from build123d import *

# Parameters (mm, degrees)
TAPPED_HOLE1_D     = 6.8
SKETCH4_W          = 9.5
SKETCH4_H          = 1.5
CUT_EXTRUDE1_DEPTH = 12


with BuildPart() as part:
    # Sketch1 → Revolve1 (revolve)
    with BuildSketch(Plane(origin=(0, 0, 0), x_dir=(0, 0, -1), z_dir=(1, 0, 0))):
        Polygon((-4.75, -13.8), (-4.75, -1.4), (-4.65, -1.4), (-4.65, -1.3), (-5.55, -1.3), (-5.55, 0), (-3.25, 0), (-3.25, -14.3), (-4.461324865, -14.3), align=None)
    revolve(axis=Axis((0, 0, 0), (0, -1, 0)))

    # Tapped Hole1 (through all)
    with Locations(Plane(origin=(0, 0, 0), x_dir=(1, 0, 0), z_dir=(0, 1, 0))):
        with Locations((0, 0)):
            Hole(TAPPED_HOLE1_D / 2)

    # Sketch4 → Cut-Extrude1 (cut)
    with BuildSketch(Plane.XZ.offset(14.3)):
        Rectangle(SKETCH4_W, SKETCH4_H)
    extrude(amount=-CUT_EXTRUDE1_DEPTH, mode=Mode.SUBTRACT)


solid = part.part
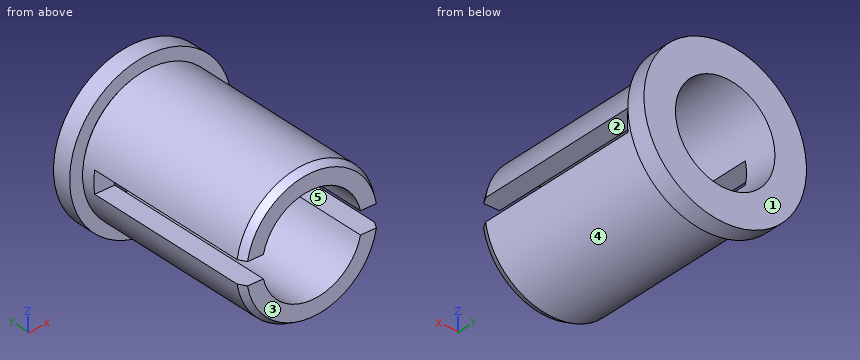
Geometry: final body of the model. Coordinates: model frame, mm. Face numbers are marked on the shaded views. A direction names the side the tool comes from. Coordinates: 2 decimals unless noted, no trailing zeros. Order: outer loops, then holes, each group sorted by start corner. A loop starts at its lowest first (then second) coordinate and runs counter-clockwise, first axis right, second up.
(1) Section query A-A (x = 0). Return the cut outline in (y, z).
(2) Draft query along Z for the marked faces 3, 4 and 5. Return one class per face: pulls with the +Z half, pulls with the -Z half, needs draft (parallel to the pull), parting line crosses it, or undercut.
(3) First-contact query: pin 1 (4 mm diameter, centred on y = -9.5, z = 2, fed in from +X); pin 2 (6 mm diameter, centred on y = -12.5, z = -3, fed in from -X); pin 3 (1.1 mm diameter, centred on x = -4, y = -8.5, fed in from -Z). Flat tips, straight axial feed; report the tip coordinate or a pass-through.
(4) Section query D-D (y = -2). Return the cut outline in (x, z).
(5) Access query for the marked faces 1 and 2. Directions: +Z, -Z, +X, -X, +Y, -Y. A direction counts if a zero-diameter tool reaches every point of the face in a straight line with its end or side. Return the directions, or none.
(6) Section query B-B (z = 0). Return the cut outline in (x, y), plus the area to 3 significant figures.
(7) Material intervals for probe 1 along Z at (x, y) = (0, -10.75); probe 2 along Z at (x, y) = (1, -4.75); probe 3 along Y at (x, z) = (-3.75, 3.25), sorted ascending.
(8) Section query C-C (y = -3.75). Return the cut outline in (x, z), plus the area to 3 significant figures.
Solution:
1. outline: (-14.3, -4.46) - (-13.8, -4.75) - (-1.4, -4.75) - (-1.4, -4.65) - (-1.3, -4.65) - (-1.3, -5.55) - (0, -5.55) - (0, -3.4) - (-14.3, -3.4) - close; (-14.3, 3.4) - (0, 3.4) - (0, 5.55) - (-1.3, 5.55) - (-1.3, 4.65) - (-1.4, 4.65) - (-1.4, 4.75) - (-13.8, 4.75) - (-14.3, 4.46) - close
2. face 3: needs draft
2. face 4: parting line crosses it
2. face 5: undercut
3. pin 1: stops at x = 4.69
3. pin 2: stops at x = -4.69
3. pin 3: stops at z = -3.26
4. outline: circle Ø9.5 at (0, 0); hole circle Ø6.8 at (0, 0)
5. face 1: +Z, -Z, +X, -X, +Y
5. face 2: +X, -X, -Y
6. outline: (-5.55, -1.3) - (-4.65, -1.3) - (-4.65, -1.4) - (-4.75, -1.4) - (-4.75, -2.3) - (-3.4, -2.3) - (-3.4, 0) - (-5.55, 0) - close; (3.4, -2.3) - (4.75, -2.3) - (4.75, -1.4) - (4.65, -1.4) - (4.65, -1.3) - (5.55, -1.3) - (5.55, 0) - (3.4, 0) - close
6. area: 8.27 mm2
7. probe 1: z = -4.75 to -3.4, 3.4 to 4.75
7. probe 2: z = -4.64 to -3.25, 3.25 to 4.64
7. probe 3: y = -1.3 to 0
8. outline: (-4.69, -0.75) arc R4.75 ccw to (4.69, -0.75) - (3.32, -0.75) arc R3.4 cw to (-3.32, -0.75) - close; (-4.69, 0.75) - (-3.32, 0.75) arc R3.4 cw to (3.32, 0.75) - (4.69, 0.75) arc R4.75 ccw to start
8. area: 30.5 mm2
